```python
from build123d import *

# Parameters (mm, degrees)
BASEHEAD_DEPTH = 13
BEARINGSKE_W   = 0.8
BEARINGSKE_H   = 2.320508076


with BuildPart() as part:
    # HeadSke → BaseHead (new body)
    with BuildSketch(Plane(origin=(0, 0, 0), x_dir=(0, 0, -1), z_dir=(1, 0, 0))):
        Polygon((15, 8.660254038), (15, -8.660254038), (0, -17.320508076), (-15, -8.660254038), (-15, 8.660254038), (0, 17.320508076), align=None)
    extrude(amount=BASEHEAD_DEPTH)

    # BodySke → BaseBody (revolve)
    with BuildSketch(Plane.XY, mode=Mode.PRIVATE) as basebody_sk:
        Polygon((0, 10.5), (0, 0), (163, 0), (163, 8.626), (161.626, 10), (139.25, 10), (137.383974596, 10.5), align=None)
    revolve(basebody_sk.sketch.rotate(Axis((0, 0, 0), (1, 0, 0)), 90), axis=Axis((0, 0, 0), (1, 0, 0)))

    # Sketch3 → HeadChamfer (revolve, cut)
    with BuildSketch(Plane(origin=(0, 0, 0), x_dir=(1, 0, 0), z_dir=(0, 1, 0))):
        Polygon((3.75, 21.495190528), (-3.75, 8.504809472), (-13.695781038, 14.247008831), (-6.195781038, 27.237389888), align=None)
    revolve(axis=Axis((0, 0, 0), (1, 0, 0)), mode=Mode.SUBTRACT)

    # BearingSke → BearingFace (revolve, cut)
    with BuildSketch(Plane.XY, mode=Mode.PRIVATE) as bearingface_sk:
        with Locations((12.6, 16.160254038)):
            Rectangle(BEARINGSKE_W, BEARINGSKE_H)
    revolve(bearingface_sk.sketch.rotate(Axis((0, 0, 0), (1, 0, 0)), 270), axis=Axis((0, 0, 0), (1, 0, 0)), mode=Mode.SUBTRACT)


solid = part.part
```
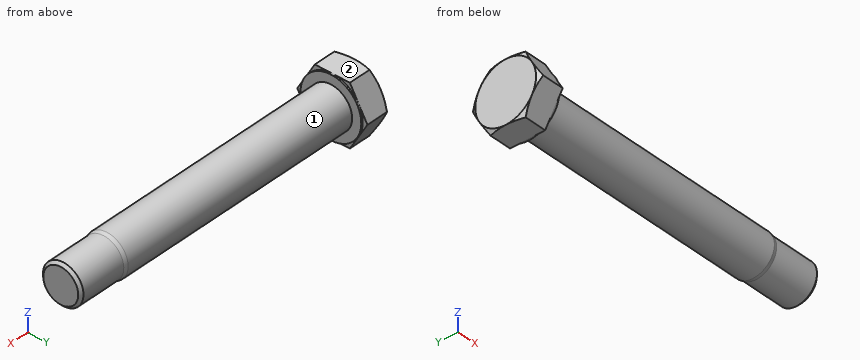
The listing builds one solid part. Answer for the finished solid, in the listing's coordinates (mm). Face numbers are marked on the shaded views. A direction names the side the tool comes from. Coordinates: 2 decimals unless noted, no trailing zeros. Write each loop counter-clockwise with the first axis right and the second up, starting at its lowest first coordinate (ties: lowest second). Pieces come first, ordered by that corner, then holes. Notation, with made-up numbers: (75, 72) - (122, 72) arc R19 cw to (122, 84) - close; hole circle Ø7 at (17, 67). An arc over 180 degrees is marked (long way). Return JSON: item names as keys, results as strings. Group by question number.
Q1. Find the intervals of material crossed by line 1 along Y through (x, z) = (82, 6); line 2 along Y through (x, z) = (52, 0); line 3 along Z through (x, y) = (114, 0.5), in increasing order. Write a range as [from, to].
Q2. The part is cut by section A-A on x = 68.5. Write down the section's boundary in (y, z), and give its area (3 significant figures).
Q3. Which of the six approach directions +Z, -Z, +X, -X, +Y, -Y give full straight-line access (tool end or side, diameter ignored) to the marked faces 1 and 2?
Q4. Flat-ended cylindrical pins translate along their axes: pin 1 Ø1 at (x, y) = (70.5, 0) entering from +Z; pin 2 Ø5 at (x, y) = (60.5, -5.5) entering from +Z; pin 3 Ø10 at (x, y) = (68, -12.5) entering from +Z. Find the tip coordinate at first contact, or state that the pin passes through.
Evaluation:
{
 "1": {"line 1": "y = [-8.62, 8.62]", "line 2": "y = [-10.5, 10.5]", "line 3": "z = [-10.49, 10.49]"},
 "2": {"outline": "circle Ø21 at (0, 0)", "area": "346 mm2"},
 "3": {"face 1": "+X", "face 2": "+Z, +X, -X, +Y, -Y"},
 "4": {"pin 1": "stops at z = 10.5", "pin 2": "stops at z = 10.06", "pin 3": "stops at z = 7.35"}
}
